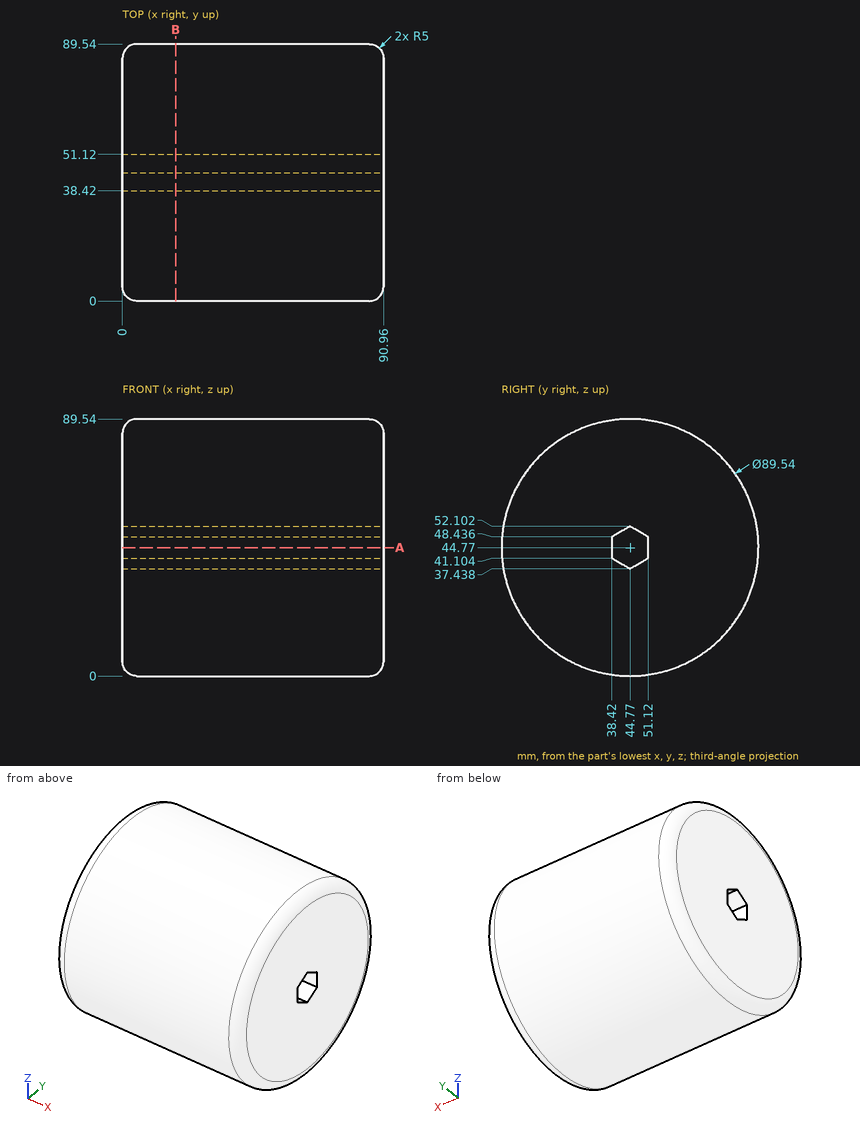
Print and shaded views of the part. All mm, measured from the part's lowest x, y and z. Coordinates: 2 decimals unless noted, no trailing zeros. Loops run counter-clockwise (first coordinate to the right, second up) from the corner with the lowest first, then second, coordinate; pieces in that order, holes last. Notation, with made-up numbers: (69, 11.25) - (84, 11.25) arc R25 cw to (84, 23.25) - close; hole circle Ø9 at (25, 27). An arc over 180 degrees is marked (long way). Use one line per item in the form item = value. Start each with the question number.
1) Flat gauge pins, fed straight in: pin 1 (2 mm diameter, centred on x = 43, z = 46.5, fed in from +Y); pin 2 (2 mm diameter, centred on x = 69, z = 14.5, fed in from +Y); pin 3 (1.5 mm diameter, centred on x = 53, z = 10.5, fed in from +Y). Where does each tip first touch, or does it go through?
2) Band-saw the part on B-B (x = 18.5). Give the cut face in (y, z), and give its area (3 significant figures).
3) Drill centre lines: L1, parallel to Z at x = 78.5, y = 51 (1 decimal); L2, parallel to Y at x = 18.5, z = 40 (1 decimal); L3, parallel to Y at x = 19.5, z = 49 (1 decimal). Where is each one in solid material? Low to high. Write a range as from..to.
4) Band-saw the part on A-A (z = 44.77). Give the cut face in (x, y), and give its area (3 significant figures).
Check values:
q1.pin_1 = 89.53
q1.pin_2 = 78.65
q1.pin_3 = 74.45
q2.outline = circle Ø89.54 at (44.77, 44.77); hole (38.42, 41.1) - (44.77, 37.44) - (51.12, 41.1) - (51.12, 48.44) - (44.77, 52.1) - (38.42, 48.44) - close
q2.area = 6,160 mm2
q3.L1 = 0.4..41, 48.5..89.1
q3.L2 = 0.3..40.3, 49.2..89.3
q3.L3 = 0.2..39.4, 50.1..89.3
q4.outline = (0, 5) arc R5 ccw to (5, 0) - (85.96, 0) arc R5 ccw to (90.96, 5) - (90.96, 38.42) - (0, 38.42) - close; (0, 51.12) - (90.96, 51.12) - (90.96, 84.54) arc R5 ccw to (85.96, 89.54) - (5, 89.54) arc R5 ccw to (0, 84.54) - close
q4.area = 6,970 mm2
